```python
from build123d import *

# Parameters (mm, degrees)
F0_R     = 3.175
F0_W     = 5.842
F0_H     = 12.7
F1_DEPTH = 6.35


with BuildPart() as f1:
    # F0 (on Front) → F1 (new body)
    with BuildSketch(Plane.XZ):
        with BuildLine():
            Line((5.842, 0), (0, 0))
            Line((0, 0), (-0.9398, 0))
            ThreePointArc((-0.9398, 0), (-3.195791, -4.549339), (-8.182663, -5.506983))
            Line((-8.182663, -5.506983), (5.842, -9.398))
            Line((5.842, -9.398), (5.842, 0))
        make_face()
        with BuildLine():
            ThreePointArc((-8.182663, -5.506983), (-3.195791, -4.549339), (-0.9398, 0))
            ThreePointArc((-0.9398, 0), (-4.591961, 5.329721), (-10.88063, 3.847543))
            ThreePointArc((-10.88063, 3.847543), (-12.145978, -1.583727), (-8.182663, -5.506983))
        make_face()
        with Locations((-6.6548, 0)):
            Circle(F0_R, mode=Mode.SUBTRACT)
        with BuildLine():
            Line((-0.9398, 0), (0, 0))
            Line((0, 0), (0, 12.7))
            Line((0, 12.7), (5.842, 12.7))
            Line((5.842, 12.7), (5.842, 15.24))
            Line((5.842, 15.24), (-0.508, 15.24))
            Line((-0.508, 15.24), (-10.88063, 3.847543))
            ThreePointArc((-10.88063, 3.847543), (-4.591961, 5.329721), (-0.9398, 0))
        make_face()
        with Locations((2.921, 6.35)):
            Rectangle(F0_W, F0_H)
        Polygon((5.842, 12.7), (5.842, 0), (66.294, 0), (66.294, 12.7), (56.134, 12.7), (56.134, 10.16), (10.16, 10.16), (10.16, 12.7), align=None)
    extrude(amount=F1_DEPTH)


solid = f1.part
```
Geometry: final body of the model. Coordinates: model frame, mm. A direction names the side the tool comes from. Coordinates: 2 decimals unless noted, no trailing zeros. Order: outer loops, then holes, each group sorted by start corner. A loop starts at its lowest first (then second) coordinate and runs counter-clockwise, first axis right, second up.
Item 1: Section query A-A (z = 1.5). Output: boundary loops of the cut face in (x, y), then the cut area to 3 significant figures.
Answer:
outline: (-12.17, -6.35) - (-9.45, -6.35) - (-9.45, 0) - (-12.17, 0) - close; (-3.86, -6.35) - (66.29, -6.35) - (66.29, 0) - (-3.86, 0) - close
area: 463 mm2
Item 2: Section query D-D (z = 7.75). Output: boundary loops of the cut face in (x, y), then the cut area to 3 significant figures.
Answer:
outline: (-7.33, -6.35) - (66.29, -6.35) - (66.29, 0) - (-7.33, 0) - close
area: 467 mm2
Item 3: Section query C-C (x = 59.5). Output: boundary loops of the cut face in (y, z).
Answer:
outline: (-6.35, 0) - (0, 0) - (0, 12.7) - (-6.35, 12.7) - close
Item 4: Access query for faces 1 (the face through (5.842, -3, -5)), 2 (the face through (10.16, -3, 11)), 3 (the face through (-3.626, -3.131, 0.954)), 4 (the face through (3, -3, 15.24)), 5 (the face through (5.842, -3, 14)). Directions: +Z, -Z, +X, -X, +Y, -Y. A direction counts if a zero-diameter tool reaches every point of the face in a straight line with its end or side. Return the directions, or none.
Answer:
face 1: -Z, +X, +Y, -Y
face 2: +Z, +Y, -Y
face 3: +Y, -Y
face 4: +Z, +X, -X, +Y, -Y
face 5: +Z, +X, +Y, -Y
Item 5: Draft query along X for faces 6 (the face through (33, -3, 10.16)), 7 (the face through (61, -3, 12.7)), 8 (the face through (-12.168, -3.131, -1.505)). Return one class per face: released by +X, released by -X, zero draft, split by the parting line, or undercut.
Answer:
face 6: undercut
face 7: zero draft
face 8: released by -X
Item 6: Section query B-B (y = -4.5). Output: boundary loops of the cut face in (x, z) (3 decimals), then the cut area to 3 significant figures.
Answer:
outline: (-10.881, 3.848) arc R5.715 ccw to (-8.183, -5.507) - (5.842, -9.398) - (5.842, 0) - (66.294, 0) - (66.294, 12.7) - (56.134, 12.7) - (56.134, 10.16) - (10.16, 10.16) - (10.16, 12.7) - (5.842, 12.7) - (5.842, 15.24) - (-0.508, 15.24) - close; hole circle Ø6.35 at (-6.655, 0)
area: 941 mm2
Item 7: Contact query for flat-ended pins moving along their axis: P1, Ø2, axis at x = 19, z = 2.5, coming from the +Y side; P2, Ø0.8, axis at y = -2.5, z = 11, coming from the -X side; P3, Ø3, axis at x = 62, y = -1.5, coming from the +Z side; P4, Ø3, axis at y = -3.5, z = -3.5, coming from the +X side. Output: stop coordinate, or through.
Answer:
P1: stops at y = 0
P2: stops at x = -4.73
P3: stops at z = 12.7
P4: stops at x = 5.84
Item 8: Material intervals for line 1 along Z through (x, y) = (46, -1.25); line 2 along Z through (x, y) = (59.5, -4.75); line 3 along X through (y, z) = (-1, -0.25), sorted ascending.
Answer:
line 1: z = 0 to 10.16
line 2: z = 0 to 12.7
line 3: x = -12.36 to -9.82, -3.49 to 5.84
